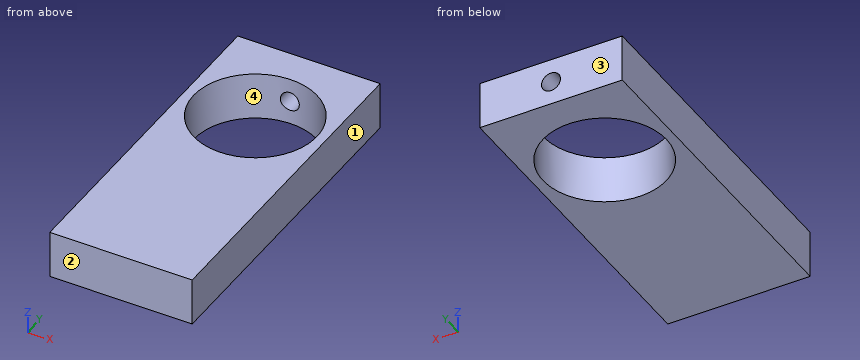
from build123d import *

# Parameters (mm, degrees)
SKETCH1_W           = 15
SKETCH1_H           = 35
BOSS_EXTRUDE1_DEPTH = 5
SKETCH2_R           = 6.5
CUT_EXTRUDE1_DEPTH  = 5
CUT_EXTRUDE2_REACH  = 37
SKETCH3_R           = 1


with BuildPart() as part:
    # Sketch1 → Boss-Extrude1 (new body)
    with BuildSketch(Plane.XY):
        with Locations((4.397758993, 4.909943839)):
            Rectangle(SKETCH1_W, SKETCH1_H)
    extrude(amount=BOSS_EXTRUDE1_DEPTH)

    # Sketch2 → Cut-Extrude1 (cut)
    with BuildSketch(Plane(origin=(0, 0, 0), x_dir=(-1, 0, 0), z_dir=(0, 0, -1))):
        with Locations((-4.397758993, 12.409943839)):
            Circle(SKETCH2_R)
    extrude(amount=-CUT_EXTRUDE1_DEPTH, mode=Mode.SUBTRACT)

    # Sketch3 → Cut-Extrude2 (cut, up to next)
    with BuildSketch(Plane(origin=(0, 22.409943839, 0), x_dir=(1, 0, 0), z_dir=(0, 1, 0)), mode=Mode.PRIVATE) as cut_extrude2_sk1:
        with Locations((4.397758993, -2.5)):
            Circle(SKETCH3_R)
    cut_extrude2_tool1 = extrude(cut_extrude2_sk1.sketch, amount=-CUT_EXTRUDE2_REACH, mode=Mode.PRIVATE) & part.part
    add(cut_extrude2_tool1.solids().sort_by_distance((4.397759, 22.409944, 2.5))[0], mode=Mode.SUBTRACT)


solid = part.part
Verification items for the finished model (mm, model axes). Face numbers are marked on the shaded views. Give positions to 0.01 mm unless a question says otherwise; leave off trailing zeros. Write each loop counter-clockwise with the first axis right and the second up, starting at its lowest first coordinate (ties: lowest second). Pieces come first, ordered by that corner, then holes.
(1) Cross-section at B-B (y = 10). Enter the section's corners in (x, z), plus the area to 3 significant figures.
(2) Cross-section at D-D (x = 4). Enter the section's corners in (y, z), plus the area to 3 significant figures.
(3) Gauge pin test, flat end, axial feed: pin 1 (1.2 mm diameter, centred on x = 4.4, z = 2.5, fed in from +Y). Record the tip position at first contact, or that the pin passes through.
(4) Cross-section at A-A (z = 2.5). Enter the section's corners in (x, y), plus the area to 3 significant figures.
(5) Mould release check, pull along Y, two halves, no side actions. Record for the marked faces 1, 2, 3 and 4: +Y half, -Y half, draft (parallel to the pull), parting line (faces both ways), or undercut.
(6) Cross-section at C-C (x = 6). Enter the section's corners in (y, z), plus the area to 3 significant figures.
(7) Material ranges on line 1 (X direction, y = 21.2, z = 2.5); line 2 (X direction, y = 13, z = 0.5); line 3 (Y direction, x = 0.25, z = 3.5), recorded low to high.
Worked out:
1. outline: (-3.1, 0) - (-1.64, 0) - (-1.64, 5) - (-3.1, 5) - close; (10.43, 0) - (11.9, 0) - (11.9, 5) - (10.43, 5) - close
1. area: 14.6 mm2
2. outline: (-12.59, 0) - (5.92, 0) - (5.92, 5) - (-12.59, 5) - close; (18.9, 0) - (22.41, 0) - (22.41, 1.58) - (18.9, 1.58) - close; (18.9, 3.42) - (22.41, 3.42) - (22.41, 5) - (18.9, 5) - close
2. area: 104 mm2
3. pin 1: stops at y = 5.94
4. outline: (-3.1, -12.59) - (11.9, -12.59) - (11.9, 22.41) - (5.4, 22.41) - (5.4, 18.83) arc R6.5 cw (long way) to (3.4, 18.83) - (3.4, 22.41) - (-3.1, 22.41) - close
4. area: 385 mm2
5. face 1: draft
5. face 2: -Y half
5. face 3: +Y half
5. face 4: undercut
6. outline: (-12.59, 0) - (6.11, 0) - (6.11, 5) - (-12.59, 5) - close; (18.71, 0) - (22.41, 0) - (22.41, 5) - (18.71, 5) - close
6. area: 112 mm2
7. line 1: x = -3.1 to 3.4, 5.4 to 11.9
7. line 2: x = -3.1 to -2.08, 10.87 to 11.9
7. line 3: y = -12.59 to 7.41, 17.41 to 22.41
